Answer from the drawing. Dimensions are ordinates in mm from the lowest x, y and z of the part. Give positions to 0.01 mm unless a question says otherwise; leave off trailing zeros. Order: outer loops, then holes, each group sorted by start corner. A loop starts at its lowest first (then second) coordinate and runs counter-clockwise, first axis right, second up. Notation, with made-up numbers: (-24, 50.5) - (-15, 50.5) arc R8 cw to (-15, 54.5) - close; hole circle Ø10 at (50.5, 19.5). An arc over 180 degrees is marked (long way). Answer in a Markdown table with one row per item.
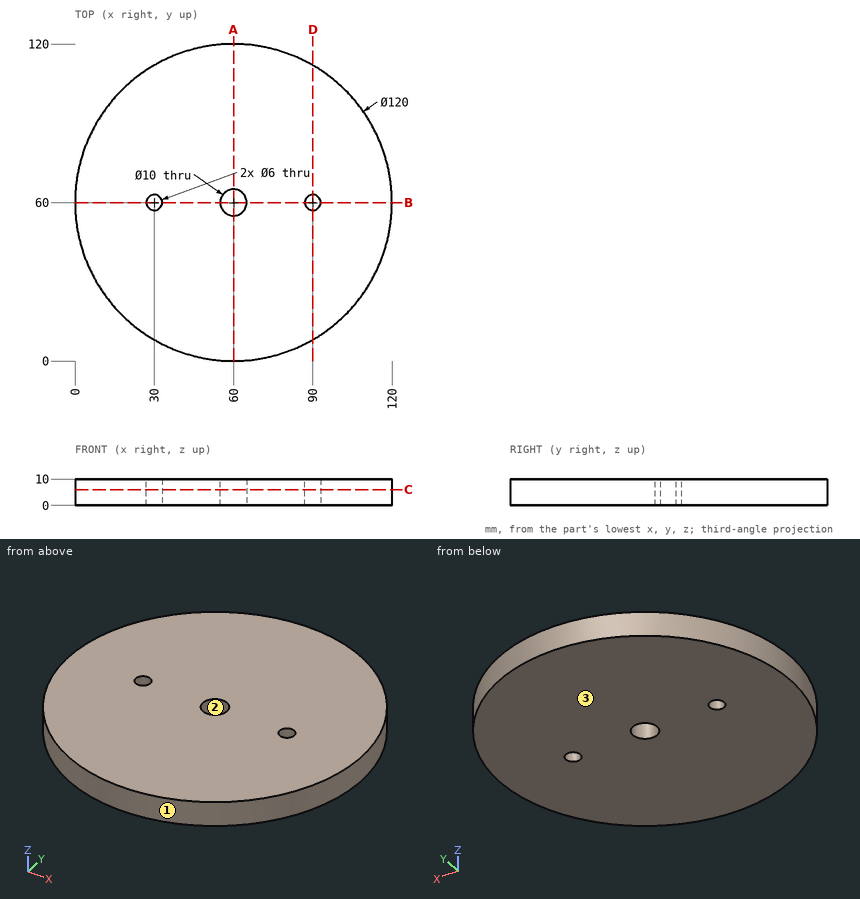
Item 1: Find section B-B on y = 60. Write down the section's boundary in (x, z).
Answer block:
| item | result |
|---|---|
| outline | (0, 0) - (27, 0) - (27, 10) - (0, 10) - close; (33, 0) - (55, 0) - (55, 10) - (33, 10) - close; (65, 0) - (87, 0) - (87, 10) - (65, 10) - close; (93, 0) - (120, 0) - (120, 10) - (93, 10) - close |
Item 2: Find section C-C on z = 6. Write down the section's boundary in (x, y).
Answer block:
| item | result |
|---|---|
| outline | circle Ø120 at (60, 60); hole circle Ø6 at (30, 60); hole circle Ø10 at (60, 60); hole circle Ø6 at (90, 60) |
Item 3: Find section A-A on x = 60. Write down the section's boundary in (y, z), then the cut area to 3 significant figures.
Answer block:
| item | result |
|---|---|
| outline | (0, 0) - (55, 0) - (55, 10) - (0, 10) - close; (65, 0) - (120, 0) - (120, 10) - (65, 10) - close |
| area | 1,100 mm² |
Item 4: Consider line 1 (Y direction, x = 60, z = 6); line 2 (Y direction, x = 30, z = 7.5); line 3 (Y direction, x = 45, z = 2). Determine where each line is inside the solid, lowest interval first.
Answer block:
| item | result |
|---|---|
| line 1 | 0 to 55, 65 to 120 |
| line 2 | 8.04 to 57, 63 to 111.96 |
| line 3 | 1.91 to 118.09 |
Item 5: Find section D-D on x = 90. Write down the section's boundary in (y, z).
Answer block:
| item | result |
|---|---|
| outline | (8.04, 0) - (57, 0) - (57, 10) - (8.04, 10) - close; (63, 0) - (111.96, 0) - (111.96, 10) - (63, 10) - close |
Item 6: Each of these flat-tipped pins is pushed along its axis until it touches: P1, Ø1, axis at y = 28.5, z = 3, coming from the +X side; P2, Ø3, axis at y = 12.5, z = 4, coming from the +X side; P3, Ø5, axis at x = 90, y = 60, coming from the -Z side; P4, Ø2, axis at y = 96, z = 1.5, coming from the -X side. Where does it stop, or does it pass through?
Answer block:
| item | result |
|---|---|
| P1 | x = 111.37 |
| P2 | x = 98.52 |
| P3 | through |
| P4 | x = 11.27 |
Item 7: Determine the mould class of the marked faces 1, 2 and 3 for opening direction Y: pulls with the +Y half, pulls with the -Y half, needs draft (parallel to the pull), parting line crosses it, or undercut.
Answer block:
| item | result |
|---|---|
| face 1 | parting line crosses it |
| face 2 | undercut |
| face 3 | needs draft |
